```python
from build123d import *

# Parameters (mm, degrees)
SKETCH_1_R                        = 4.35
EXTRUDE_1_DEPTH                   = 12
CUT_EXTRUDE_480_DEPTH             = 9
CUT_EXTRUDE_727_REACH             = 15.485
CUT_EXTRUDE_727_DIRECTION_2_REACH = 15.485


with BuildPart() as part:
    # Эскиз1 → Бобышка-Вытянуть1 (new body)
    with BuildSketch(Plane.XY):
        Circle(SKETCH_1_R)
    extrude(amount=EXTRUDE_1_DEPTH)

    # Эскиз2 → Cut-Extrude 480 (cut)
    with BuildSketch(Plane.XY.offset(12)):
        Polygon((0, 3.319764048), (-2.875, 1.659882024), (-2.875, -1.659882024), (0, -3.319764048), (2.875, -1.659882024), (2.875, 1.659882024), align=None)
    extrude(amount=-CUT_EXTRUDE_480_DEPTH, mode=Mode.SUBTRACT)

    # Эскиз3 → Cut-Extrude 727 (cut, up to next)
    with BuildSketch(Plane(origin=(0, 0, 0), x_dir=(1, 0, 0), z_dir=(0, 1, 0)), mode=Mode.PRIVATE) as cut_extrude_727_sk1:
        Polygon((-4.35, 0), (4.35, -3.166541038), (4.35, 0), align=None)
    cut_extrude_727_tool1 = extrude(cut_extrude_727_sk1.sketch, amount=-CUT_EXTRUDE_727_REACH, mode=Mode.PRIVATE) & part.part
    add(cut_extrude_727_tool1.solids().sort_by_distance((1.45, 0, 1.055514))[0], mode=Mode.SUBTRACT)

    # Эскиз3 → Cut-Extrude 727 direction 2 (cut, up to next)
    with BuildSketch(Plane(origin=(0, 0, 0), x_dir=(1, 0, 0), z_dir=(0, 1, 0)), mode=Mode.PRIVATE) as cut_extrude_727_direction_2_sk1:
        Polygon((-4.35, 0), (4.35, -3.166541038), (4.35, 0), align=None)
    cut_extrude_727_direction_2_tool1 = extrude(cut_extrude_727_direction_2_sk1.sketch, amount=CUT_EXTRUDE_727_DIRECTION_2_REACH, mode=Mode.PRIVATE) & part.part
    add(cut_extrude_727_direction_2_tool1.solids().sort_by_distance((1.45, 0, 1.055514))[0], mode=Mode.SUBTRACT)


solid = part.part
```
Here's how the part is built. I have some questions about the finished solid (model axes, mm). A direction names the side the tool comes from. Give positions to 0.01 mm unless a question says otherwise; leave off trailing zeros. Loops run counter-clockwise (first coordinate to the right, second up) from the corner with the lowest first, then second, coordinate; pieces in that order, holes last. Notation, with made-up numbers: M 45.25,62.25 L 65.25,62.25 A23 ccw 65.25,74.25 Z; hole C 30,31.25 d7. An arc over 180 degrees is marked long. Use one line per item in the form item = value. Start each with the question number.
Q1. Will these pins go through, and if not, where does the flat tip stop? pin 1 Ø2 at (x, y) = (-2.5, -0.5) entering from +Z; pin 2 Ø1.5 at (y, z) = (1, 5) entering from +X; pin 3 Ø4 at (x, z) = (2.5, 3.5) entering from -Y.
Q2. I need wall thicknesses on line 1 along Y through (x, z) = (1.5, 6); line 2 along X through (y, z) = (-2, 4.5); line 3 along X through (y, z) = (-1, 5.5) (1 decimal). Which ranges of each line are inside material? Lowest first, please.
Q3. Thinking about a two-plate mould opening in Y: for faces 3 (the flat face through (-1.458, -2.478, 7.563)), 4 (the cylindrical face through (-4.346, 0.191, 7.249)), 5 (the flat face through (-0.06, 0.06, 1.56)), which applies, +Y half, -Y half, draft (parallel to the pull), parting line (faces both ways), or undercut?
Q4. Which directions (+Z, -Z, +X, -X, +Y, -Y) give clear straight access to the entire face, cutting with the end or side of a thin tool? Please do faces 1 (the flat face through (-1, -3, 12)), 2 (the flat face through (-2.875, 0, 8)).
Q5. If we section it at C-C (x = 1.25): Write out the boundary of the cut face in (y, z), then the cut area to 3 significant figures.
Q6. If we section it at B-B (y = 0): Write out the boundary of the cut face in (x, z) (3 decimals).
Q7. If we section it at A-A (z = 8.5): Write out the boundary of the cut face in (x, y) (3 decimals).
Taken from the geometry:
q1.pin_1 = 12
q1.pin_2 = 4.34
q1.pin_3 = -4.32
q2.line_1 = -4.08 to -2.45, 2.45 to 4.08
q2.line_2 = -3.86 to -2.29, 2.29 to 3.86
q2.line_3 = -4.2 to -2.9, 2.9 to 4.2
q3.face_3 = undercut
q3.face_4 = parting line
q3.face_5 = draft
q4.face_1 = +Z, +X, -X, +Y, -Y
q4.face_2 = +Z
q5.outline = M -4.17,2.04 L 4.17,2.04 L 4.17,12 L 2.6,12 L 2.6,3 L -2.6,3 L -2.6,12 L -4.17,12 Z
q5.area = 36.2 mm^2
q6.outline = M -4.35,0 L 4.35,3.167 L 4.35,12 L 2.875,12 L 2.875,3 L -2.875,3 L -2.875,12 L -4.35,12 Z
q7.outline = C 0,0 d8.7; hole M -2.875,-1.66 L 0,-3.32 L 2.875,-1.66 L 2.875,1.66 L 0,3.32 L -2.875,1.66 Z
